Part model, mm, in its own coordinate system. Face numbers are marked on the shaded views. A direction names the side the tool comes from. Give positions to 0.01 mm unless a question says otherwise; leave off trailing zeros. Write each loop counter-clockwise with the first axis right and the second up, starting at its lowest first coordinate (ties: lowest second). Pieces come first, ordered by that corner, then holes. Notation, with made-up numbers: M 28.5,-27.75 L 79.5,-27.75 A13 ccw 79.5,-20.75 Z; hole C -9,62.5 d8. An arc over 180 degrees is marked long. Use a Markdown table: item, result.
```python
from build123d import *

# Parameters (mm, degrees)
SKETCH1_R           = 1
BOSS_EXTRUDE1_DEPTH = 5
BOSS_EXTRUDE2_DEPTH = 5
SKETCH6_W           = 20
SKETCH6_H           = 6
CUT_EXTRUDE1_DEPTH  = 5


with BuildPart() as part:
    # Sketch1 → Boss-Extrude1 (new body)
    with BuildSketch(Plane(origin=(0, 0, 0), x_dir=(1, 0, 0), z_dir=(0, 1, 0))):
        with BuildLine():
            Line((-6.063583, -8.020726268), (3.936417, -8.020726268))
            Line((3.936417, -8.020726268), (3.936417, 31.979273732))
            Line((3.936417, 31.979273732), (-6.063583, 31.979273732))
            ThreePointArc((-6.063583, 31.979273732), (-13.134650812, 29.050341544), (-16.063583, 21.979273732))
            Line((-16.063583, 21.979273732), (-16.063583, 1.979273732))
            ThreePointArc((-16.063583, 1.979273732), (-13.134650812, -5.09179408), (-6.063583, -8.020726268))
        make_face()
        with Locations((-6.063583, 21.979273732)):
            Circle(SKETCH1_R, mode=Mode.SUBTRACT)
        with Locations((-6.063583, 1.979273732)):
            Circle(SKETCH1_R, mode=Mode.SUBTRACT)
    extrude(amount=BOSS_EXTRUDE1_DEPTH)

    # Sketch5 → Boss-Extrude2 (add)
    with BuildSketch(Plane(origin=(3.936417, 0, 0), x_dir=(0, 0, -1), z_dir=(1, 0, 0))):
        Polygon((-8.020726268, 5), (31.979273732, 5), (31.979273732, 89.50779106), (19.612713583, 94.015582119), (19.612713583, 85), (4.345833881, 85), (4.345833881, 94.015582119), (-8.020726268, 89.50779106), align=None)
    extrude(amount=-BOSS_EXTRUDE2_DEPTH)

    # Sketch6 → Cut-Extrude1 (cut)
    with BuildSketch(Plane.ZY.offset(1.063583)):
        with Locations((-11.979273732, 13)):
            Rectangle(SKETCH6_W, SKETCH6_H)
    extrude(amount=-CUT_EXTRUDE1_DEPTH, mode=Mode.SUBTRACT)


solid = part.part
```
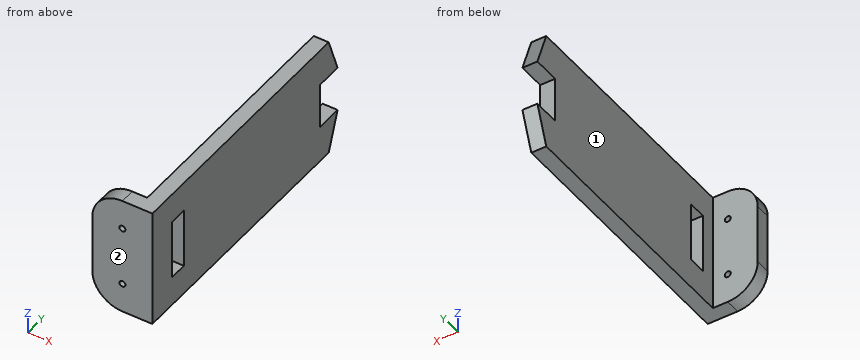
1. Cut at B-B, the plane x = 0.25. Give the cut face in (y, z), then the cut area to 3 significant figures.
Findings below:
| item | result |
|---|---|
| outline | M 0,-31.98 L 89.51,-31.98 L 94.02,-19.61 L 85,-19.61 L 85,-4.35 L 94.02,-4.35 L 89.51,8.02 L 0,8.02 Z; hole M 10,-21.98 L 16,-21.98 L 16,-1.98 L 10,-1.98 Z |
| area | 3,450 mm2 |
2. Tool access for the marked faces 1 and 2: list every direction of +Z, -Z, +X, -X, +Y, -Y with a clear straight run to the whole face (end or side of a thin tool).
Findings below:
| item | result |
|---|---|
| face 1 | +Z, -Z, -X, +Y |
| face 2 | +Z, -Z, +X, -X, -Y |
3. Cut at A-A, the plane z = -12. Give the cut face in (x, y).
Findings below:
| item | result |
|---|---|
| outline | M -16.06,0 L 3.94,0 L 3.94,10 L -1.06,10 L -1.06,5 L -16.06,5 Z; M -1.06,16 L 3.94,16 L 3.94,85 L -1.06,85 Z |
4. Cut at D-D, the plane z = 1. Give the cut face in (x, y), then the cut area to 3 significant figures.
Findings below:
| item | result |
|---|---|
| outline | M -15.61,0 L 3.94,0 L 3.94,92.07 L -1.06,92.07 L -1.06,5 L -15.61,5 Z |
| area | 533 mm2 |
5. Drill centre lines: L1, parallel to Y at x = 1.5, z = -10; L2, parallel to Y at x = -9.75, z = -11; L3, parallel to X at y = 69, z = -29. Where is each one in solid material? Low to high.
Findings below:
| item | result |
|---|---|
| L1 | 0 to 10, 16 to 85 |
| L2 | 0 to 5 |
| L3 | -1.06 to 3.94 |
6. Drop flat-ended pins along their axis: P1, Ø6, axis at x = -5, y = 82, coming from the +Z side (3 decimals); P2, Ø12, axis at x = -9, z = -17, coming from the +Y side; P3, Ø1.5, axis at x = 0.5, z = -12, coming from the +Y side; P4, Ø6, axis at x = -3, y = 16, coming from the +Z side. Give the stop position or say it passes through.
Findings below:
| item | result |
|---|---|
| P1 | through |
| P2 | y = 5 |
| P3 | y = 85 |
| P4 | z = 8.02 |
7. Cut at C-C, the plane y = 56.5. Give the cut face in (x, z), then the cut area to 3 significant figures.
Findings below:
| item | result |
|---|---|
| outline | M -1.06,-31.98 L 3.94,-31.98 L 3.94,8.02 L -1.06,8.02 Z |
| area | 200 mm2 |
